For this review, take the finished solid that the model builds, in its own axes (mm). A direction names the side the tool comes from. Round coordinates to 2 decimals unless told otherwise and drop trailing zeros. Order: outer loops, then holes, each group sorted by start corner. A loop starts at its lowest first (then second) coordinate and runs counter-clockwise, first axis right, second up. Notation, with made-up numbers: (-16, 32.5) - (11, 32.5) arc R34 ccw to (11, 69.5) - close; hole circle Ø8 at (-25.5, -38.75). An arc over 180 degrees is marked (long way). Write each question's results on one line, items separated by ' | '. Start each with the question number.
(1) Take a section at A-A, the plane z = -16. Give the boundary of the cut face in (x, y), plus the area to 3 significant figures.
(2) Take a section at B-B, the plane y = 13. Give the boundary of the cut face in (x, z).
(3) Take a section at D-D, the plane y = -3.75. Give the boundary of the cut face in (x, z), plus the area to 3 significant figures.
(4) For faces 5 (the flat face through (-34.4, 14.5, -6.656)), 6 (the flat face through (-22.327, -7, -17)), 7 (the flat face through (-21, -2.4, -17)), 8 (the flat face through (-49, -6, -12.156)), list the 3-axis set-ups (+Z, -Z, +X, -X, +Y, -Y) from which the entire face can be reached by the end or side of a thin tool; tool diameter is ignored.
(5) For L1, parallel to Z at x = -43, y = 9.5; L2, parallel to X at y = 6.25, z = -13.5; L3, parallel to X at y = 13.75, z = 12.5, list the stretches that pass through material, from the lowest coordinate up. Write a range as from..to.
(6) Insertion check: pin 1 Ø9 at (x, z) = (-36.5, 2.5) entering from +Y; pin 2 Ø0.6 at (x, y) = (-47.5, -6) entering from +Z; pin 3 Ø5 at (x, y) = (-38, 0.5) entering from -Z; pin 4 Ø1.7 at (x, z) = (-21.5, -17.5) entering from +Y. Each pin has a flat end and moves straight along its axis. Give the tip position at first contact, or say it passes through.
(7) Draft analysis for pull direction X (two halves, no side actions). For faces 1 (the flat face through (-49, -11.5, -16)), 2 (the flat face through (-50.69, 7, 3)), 3 (the flat face through (-17.69, 5, -1)), 4 (the flat face through (-47, -7, -15.278)), state which applies: pulls with the +X half, pulls with the -X half, needs draft (parallel to the pull), parting line crosses it, or undercut.
(8) Take a section at C-C, the plane x = -43. Give the boundary of the cut face in (y, z), plus the area to 4 significant figures.
```python
from build123d import *

# Parameters (mm, degrees)
SKETCH_1_W          = 33
SKETCH_1_H          = 38
SKETCH_1_W_2        = 27.5
SKETCH_1_H_2        = 29.5
EXTRUDE_1_DEPTH     = 15
SKETCH_1_3_W        = 27.5
SKETCH_1_3_H        = 29.5
SKETCH_1_3_W_2      = 16
SKETCH_1_3_H_2      = 26.5
EXTRUDE_2_DEPTH     = 2
SKETCH_2_W          = 29.5
SKETCH_2_H          = 31.5
CUT_EXTRUDE_1_DEPTH = 1
SKETCH_3_W          = 11.060472634
SKETCH_3_H          = 5.5
EXTRUDE_3_DEPTH     = 11.5
EXTRUDE_4_DEPTH     = 9.1
SKETCH_5_W          = 2.491276019
SKETCH_5_H          = 6.268810469
EXTRUDE_5_DEPTH     = 17.4
SKETCH_6_W          = 2.530660276
SKETCH_6_H          = 6.244059343
EXTRUDE_6_DEPTH     = 26.5
SKETCH_6_3_W        = 2.054656533
SKETCH_6_3_H        = 3.122029671
EXTRUDE_7_DEPTH     = 9.1


with BuildPart() as part:
    # Sketch 1 → Extrude 1 (new body)
    with BuildSketch(Plane(origin=(0, 0, 0), x_dir=(1, 0, 0), z_dir=(0, 1, 0))):
        with Locations((-34.189708408, -6.844356319)):
            Rectangle(SKETCH_1_W, SKETCH_1_H)
        with Locations((-34.180787321, -9.094356319)):
            Rectangle(SKETCH_1_W_2, SKETCH_1_H_2, mode=Mode.SUBTRACT)
    extrude(amount=EXTRUDE_1_DEPTH)

    # Sketch 1_3 → Extrude 2 (add)
    with BuildSketch(Plane(origin=(0, 0, 0), x_dir=(1, 0, 0), z_dir=(0, 1, 0))):
        with Locations((-34.180787321, -9.094356319)):
            Rectangle(SKETCH_1_3_W, SKETCH_1_3_H)
        with Locations((-38.930787321, -8.594356319)):
            Rectangle(SKETCH_1_3_W_2, SKETCH_1_3_H_2, mode=Mode.SUBTRACT)
        Polygon((-26.430787321, -11.844851054), (-26.430787321, -15.844356319), (-29.430787321, -15.844356319), (-29.43078728, -11.844356319), align=None, mode=Mode.SUBTRACT)
    extrude(amount=EXTRUDE_2_DEPTH)

    # Sketch 2 → Cut-Extrude 1 (cut)
    with BuildSketch(Plane(origin=(0, 15, 0), x_dir=(1, 0, 0), z_dir=(0, 1, 0))):
        with Locations((-34.180787321, -9.094356319)):
            Rectangle(SKETCH_2_W, SKETCH_2_H)
    extrude(amount=-CUT_EXTRUDE_1_DEPTH, mode=Mode.SUBTRACT)

    # Sketch 3 → Extrude 3 (add)
    with BuildSketch(Plane.XZ):
        with Locations((-23.219944725, -9.405643681)):
            Rectangle(SKETCH_3_W, SKETCH_3_H)
    extrude(amount=EXTRUDE_3_DEPTH)

    # Sketch 4 → Extrude 4 (add)
    with BuildSketch(Plane.XZ.offset(11.5)):
        Polygon((-17.689708408, -12.155643681), (-20.180984427, -12.155643681), (-20.180984427, -15.342965437), (-22.327356321, -15.342965437), (-22.327356321, -18.42445415), (-20.180984427, -18.42445415), (-17.689708408, -18.42445415), align=None)
    extrude(amount=-EXTRUDE_4_DEPTH)

    # Sketch 5 → Extrude 5 (add)
    with BuildSketch(Plane(origin=(0, -2.4, 0), x_dir=(1, 0, 0), z_dir=(0, 1, 0))):
        with Locations((-18.935346417, 15.290048916)):
            Rectangle(SKETCH_5_W, SKETCH_5_H)
    extrude(amount=EXTRUDE_5_DEPTH)

    # Sketch 6 → Extrude 6 (add)
    with BuildSketch(Plane.XZ.offset(11.5)):
        with Locations((-49.42437827, -15.277673353)):
            Rectangle(SKETCH_6_W, SKETCH_6_H)
    extrude(amount=-EXTRUDE_6_DEPTH)

    # Sketch 6_3 → Extrude 7 (add)
    with BuildSketch(Plane.XZ.offset(11.5)):
        with Locations((-47.131719866, -16.838688189)):
            Rectangle(SKETCH_6_3_W, SKETCH_6_3_H)
    extrude(amount=-EXTRUDE_7_DEPTH)


solid = part.part
```
Results below:
1) outline: (-50.69, -11.5) - (-46.1, -11.5) - (-46.1, -2.4) - (-48.16, -2.4) - (-48.16, 15) - (-50.69, 15) - close; (-22.33, -11.5) - (-17.69, -11.5) - (-17.69, 15) - (-20.18, 15) - (-20.18, -2.4) - (-22.33, -2.4) - close | area: 171 mm^2
2) outline: (-50.69, -18.4) - (-48.16, -18.4) - (-48.16, -12.16) - (-20.18, -12.16) - (-20.18, -18.42) - (-17.69, -18.42) - (-17.69, 25.84) - (-50.69, 25.84) - close; hole (-47.93, -5.66) - (-20.43, -5.66) - (-20.43, 23.84) - (-47.93, 23.84) - close
3) outline: (-50.69, -18.4) - (-46.1, -18.4) - (-46.1, -15.28) - (-48.16, -15.28) - (-48.16, -12.16) - (-50.69, -12.16) - close; (-28.75, -12.16) - (-20.18, -12.16) - (-20.18, -15.34) - (-22.33, -15.34) - (-22.33, -18.42) - (-17.69, -18.42) - (-17.69, -6.66) - (-28.75, -6.66) - close | area: 105 mm^2
4) face 5: +Y | face 6: -Z, +Y, -Y | face 7: -Z, +Y | face 8: +Z, -X, -Y
5) L1: z = -12.16..-5.66, 23.84..25.84 | L2: x = -50.69..-48.16, -20.18..-17.69 | L3: x = -50.69..-47.93, -20.43..-17.69
6) pin 1: passes through | pin 2: stops at z = -15.28 | pin 3: stops at z = -12.16 | pin 4: stops at y = -2.4
7) face 1: needs draft | face 2: pulls with the -X half | face 3: pulls with the +X half | face 4: undercut
8) outline: (0, -12.16) - (15, -12.16) - (15, -6.66) - (14, -6.66) - (14, -5.66) - (2, -5.66) - (2, -4.66) - (0, -4.66) - close; (0, 21.84) - (2, 21.84) - (2, 23.84) - (14, 23.84) - (14, 24.84) - (15, 24.84) - (15, 25.84) - (0, 25.84) - close | area: 131.5 mm^2
